```python
from build123d import *

# Parameters (mm, degrees)
SKETCH1_R           = 4.8
BOSS_EXTRUDE2_DEPTH = 32
SKETCH2_R           = 2.95
BOSS_EXTRUDE3_DEPTH = 16
BOSS_EXTRUDE4_START = 16
SKETCH3_R           = 2.95
BOSS_EXTRUDE4_DEPTH = 16
FILLET1_R           = 1
SKETCH4_R           = 7
BOSS_EXTRUDE5_DEPTH = 0.4


with BuildPart() as part:
    # Sketch1 → Boss-Extrude2 (new body)
    with BuildSketch(Plane(origin=(0, 0, 0), x_dir=(1, 0, 0), z_dir=(0, 1, 0))):
        with Locations(Location((0, 0, 0), (0, 0, 270))):
            Circle(SKETCH1_R)
    extrude(amount=BOSS_EXTRUDE2_DEPTH)

    # Sketch2 → Boss-Extrude3 (add)
    with BuildSketch(Plane(origin=(0, 32, 0), x_dir=(1, 0, 0), z_dir=(0, 1, 0))):
        with Locations(Location((0, 0, 0), (0, 0, 270))):
            Circle(SKETCH2_R)
    extrude(amount=BOSS_EXTRUDE3_DEPTH)

    # Sketch3 → Boss-Extrude4 (add)
    with BuildSketch(Plane.XZ.offset(BOSS_EXTRUDE4_START)):
        with Locations(Location((0, 0, 0), (0, 0, 90))):
            Circle(SKETCH3_R)
    extrude(amount=-BOSS_EXTRUDE4_DEPTH)

    # Fillet1
    fillet1_edges = [part.edges().sort_by_distance(p)[0] for p in [
        (0, 0, -4.8),
        (0, 32, -4.8),
    ]]
    fillet(fillet1_edges, radius=FILLET1_R)

    # Sketch4 → Boss-Extrude5 (add)
    with BuildSketch(Plane(origin=(0, 48, 0), x_dir=(1, 0, 0), z_dir=(0, 1, 0))):
        with Locations(Location((0, 0, 0), (0, 0, 270))):
            Circle(SKETCH4_R)
    extrude(amount=BOSS_EXTRUDE5_DEPTH)


solid = part.part
```
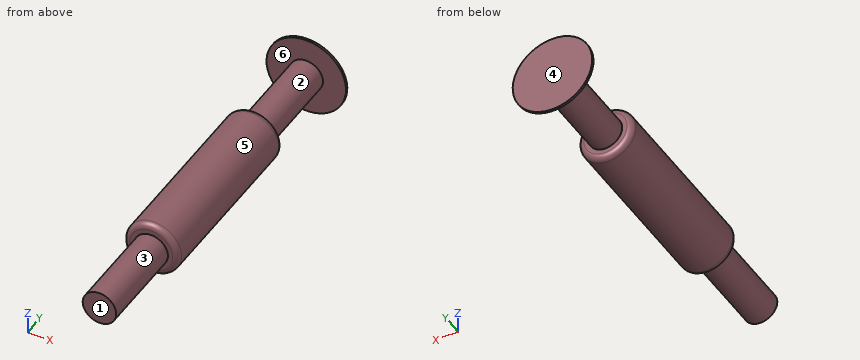
Source: CAD feature listing. Evaluate the final solid. Frame: model axes, mm. Face numbers are marked on the shaded views. A direction names the side the tool comes from. Give positions to 0.01 mm unless a question says otherwise; leave off trailing zeros. Loops run counter-clockwise (first coordinate to the right, second up) from the corner with the lowest first, then second, coordinate; pieces in that order, holes last. Notation, with made-up numbers: M 84,72.5 L 105,72.5 A24 cw 105,97.5 Z; hole C -34,-36 d9. An arc over 180 degrees is marked long. Put each result on its own line as item: value.
Q1. Pin query (flat end, axial travel): P1, Ø6, axis at x = -3.5, y = 6.5, coming from the -Z side; P2, Ø1, axis at x = -2.5, y = 22, coming from the +Z side; P3, Ø2, axis at y = 3, z = 3, coming from the -X side. Return the tip coordinate at first contact, or that it passes through.
Response values:
P1: stops at z = -4.77
P2: stops at z = 4.36
P3: stops at x = -4.36
Q2. Mould query, pull axis Y, two halves, no side actions, for the marked faces 4, 5 and 6. Classes: released by +Y, released by -Y, zero draft, split by the parting line, or undercut.
Response values:
face 4: released by +Y
face 5: zero draft
face 6: undercut
Q3. Section D-D (y = 27.5). Return the cut outline in (x, z), and give its area (3 significant figures).
Response values:
outline: C 0,0 d9.6
area: 72.4 mm²
Q4. Section A-A (x = 0). Return the cut outline in (y, z).
Response values:
outline: M -16,-2.95 L 0,-2.95 L 0,-3.8 A1 ccw 1,-4.8 L 31,-4.8 A1 ccw 32,-3.8 L 32,-2.95 L 48,-2.95 L 48,-7 L 48.4,-7 L 48.4,7 L 48,7 L 48,2.95 L 32,2.95 L 32,3.8 A1 ccw 31,4.8 L 1,4.8 A1 ccw 0,3.8 L 0,2.95 L -16,2.95 Z
Q5. Section B-B (z = 0). Return the cut outline in (x, y).
Response values:
outline: M -7,48 L -2.95,48 L -2.95,32 L -3.8,32 A1 ccw -4.8,31 L -4.8,1 A1 ccw -3.8,0 L -2.95,0 L -2.95,-16 L 2.95,-16 L 2.95,0 L 3.8,0 A1 ccw 4.8,1 L 4.8,31 A1 ccw 3.8,32 L 2.95,32 L 2.95,48 L 7,48 L 7,48.4 L -7,48.4 Z
Q6. Section C-C (y = 43.5). Return the cut outline in (x, z), and give its area (3 significant figures).
Response values:
outline: C 0,0 d5.9
area: 27.3 mm²
Q7. Reachability of the marked faces 1, 2 and 3 from +Z, -Z, +X, -X, +Y, -Y: full face, straight path, thin tool, end or side. Return the list, or none.
Response values:
face 1: +Z, -Z, +X, -X, -Y
face 2: none
face 3: -Y
Q8. Line query: probe 1 along Y at (x, z) = (-1.5, 3); probe 2 along Y at (x, z) = (-4.5, 3.5); probe 3 along Y at (x, z) = (-3.75, -2.25). Output: solid intervals per line, ascending. Write a range as [from, to].
Response values:
probe 1: y = [0, 32], [48, 48.4]
probe 2: y = [48, 48.4]
probe 3: y = [0.18, 31.82], [48, 48.4]
